Geometry check sheet. Reference: drawing and pictorial views, mm from the part's lowest x, y, z. Give positions to 0.01 mm unless a question says otherwise; leave off trailing zeros. Order: outer loops, then holes, each group sorted by start corner. A loop starts at its lowest first (then second) coordinate and runs counter-clockwise, first axis right, second up.
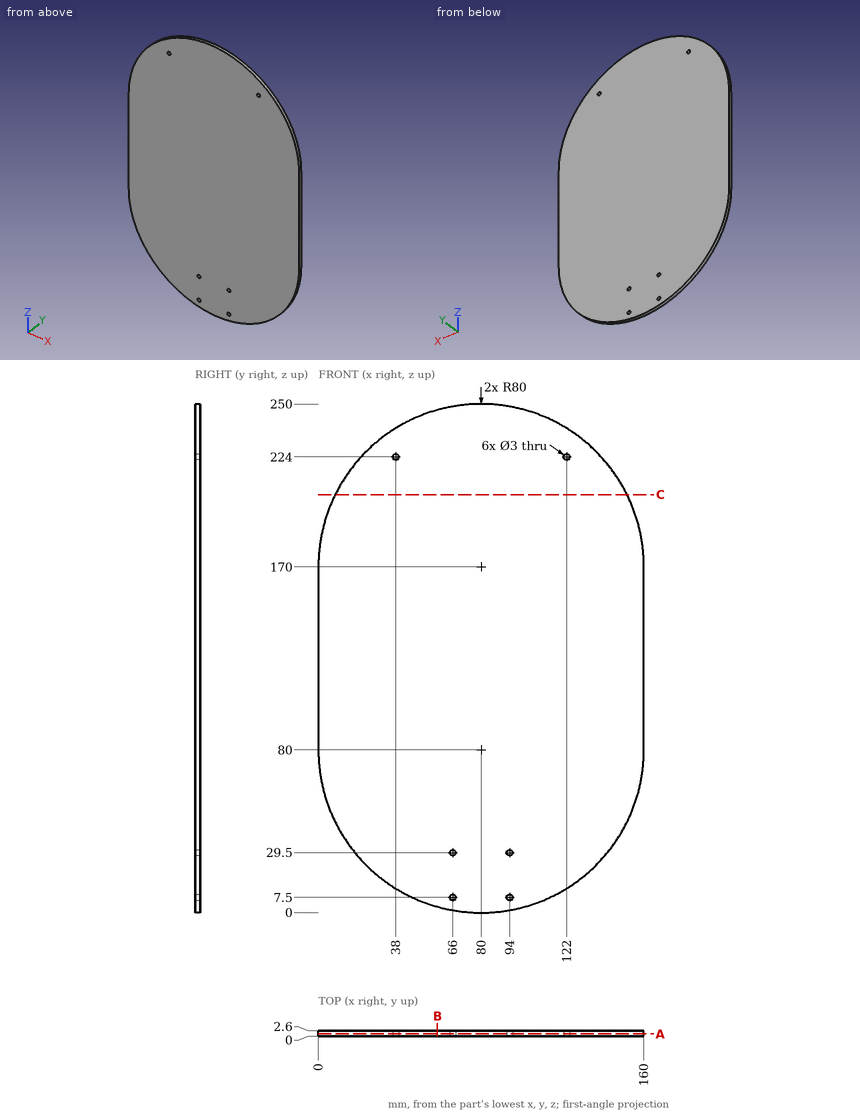
(1) Cross-section at B-B on x = 58.5. Enter the section's corners in (y, z).
Response values:
outline: (0, 2.94) - (2.6, 2.94) - (2.6, 247.06) - (0, 247.06) - close
(2) Cross-section at A-A on y = 1.1. Enter the section's corners in (x, z), then the cut area to 3 significant figures.
Response values:
outline: (0, 80) arc R80 ccw to (160, 80) - (160, 170) arc R80 ccw to (0, 170) - close; hole circle Ø3 at (38, 224); hole circle Ø3 at (66, 7.5); hole circle Ø3 at (66, 29.5); hole circle Ø3 at (94, 7.5); hole circle Ø3 at (94, 29.5); hole circle Ø3 at (122, 224)
area: 34,500 mm2
(3) Material ranges on L1, parallel to Z at x = 94, y = 0.9; L2, parallel to Z at x = 67, y = 0.6; L3, parallel to X at y = 1.3, z = 7.5, recorded low to high.
Response values:
L1: z = 1.23 to 6, 9 to 28, 31 to 248.77
L2: z = 1.06 to 6.38, 8.62 to 28.38, 30.62 to 248.94
L3: x = 46.18 to 64.5, 67.5 to 92.5, 95.5 to 113.82
(4) Cross-section at C-C on z = 205.5. Enter the section's corners in (x, y).
Response values:
outline: (8.31, 0) - (151.69, 0) - (151.69, 2.6) - (8.31, 2.6) - close
(5) Gauge pin test, flat end, axial feed: pin 1 Ø1 at (x, y) = (62, 2.5) entering from -Z. Record the tip position at first contact, or that the pin passes through.
Response values:
pin 1: stops at z = 1.94
